Source: CAD feature listing. Evaluate the final solid. Frame: model axes, mm. Give positions to 0.01 mm unless a question says otherwise; leave off trailing zeros. Write each loop counter-clockwise with the first axis right and the second up, starting at its lowest first coordinate (ties: lowest second). Pieces come first, ordered by that corner, then holes. Notation, with made-up numbers: (2.25, 28) -> (57.25, 28) arc R20 ccw to (57.25, 58) -> close; hole circle Ø11 at (89, 77). An arc over 180 degrees is marked (long way). Use one line per item in the form item = value. Start each with the question number.
(1) First-contact query: P1, Ø2, axis at x = 12.5, y = 18.5, coming from the -Z side. Flat tip, straight axial feed; report the tip coordinate or a pass-through.
(2) Cut plane B-B, the plane y = 19.1. Output: boundary loops of the cut face in (x, z).
(3) Material intervals for line 1 along Z through (x, y) = (31, 19.1); line 2 along Z through (x, y) = (39, 17.95); line 3 along X through (y, z) = (17.15, 29), sorted ascending. Write a range as from..to.
(4) Cut plane C-C, the plane z = 13. Output: boundary loops of the cut face in (x, y).
(5) Cut plane D-D, the plane z = 24.5. Output: boundary loops of the cut face in (x, y), and give its area (3 significant figures).
(6) Cut plane A-A, the plane x = 31. Output: boundary loops of the cut face in (y, z), and give its area (3 significant figures).
(7) Draft query along Z for faces 1 (the face through (14, 20, 8)), 2 (the face through (36.802, 17.972, 3.903)), 3 (the face through (7.497, 17.972, 37.787)). Return one class per face: pulls with the +Z half, pulls with the -Z half, needs draft (parallel to the pull), parting line crosses it, or undercut.
from build123d import *

# Parameters (mm, degrees)
CYLINDER019_R          = 2.2
CYLINDER019_DEPTH      = 26
CYLINDER019_ROLL_ANGLE = -90
ARRAY005_X_COUNT       = 2
ARRAY005_X_PITCH       = 8
ARRAY005_Z_COUNT       = 2
ARRAY005_Z_PITCH       = 9
CYLINDER018_R          = 30
CYLINDER018_DEPTH      = 4
CYLINDER018_ROLL_ANGLE = -90


with BuildPart() as obj1:
    # Cylinder019 → Cylinder019 (new body)
    with BuildSketch(Plane.XY):
        Circle(CYLINDER019_R)
    extrude(amount=CYLINDER019_DEPTH)


with BuildPart() as obj1_1:
    # Cylinder019 roll: moved
    add(obj1.part.rotate(Axis((0, 0, 0), (1, 0, 0)), CYLINDER019_ROLL_ANGLE))


with BuildPart() as obj1_2:
    # Cylinder019 placement: moved
    add(obj1_1.part.moved(Location((202, 0, 4))))

    # Array005 X: obj1_2


with BuildPart() as obj1_3:
    add(obj1_2.part)
    with Locations(*[(i * ARRAY005_X_PITCH, 0, 0) for i in range(1, ARRAY005_X_COUNT)]):
        add(obj1_2.part)

    # Array005 Z: obj1_2


with BuildPart() as obj1_4:
    add(obj1_3.part)
    with Locations(*[(0, 0, i * ARRAY005_Z_PITCH) for i in range(1, ARRAY005_Z_COUNT)]):
        add(obj1_3.part)


with BuildPart() as obj2:
    # Cylinder018 → Cylinder018 (new body)
    with BuildSketch(Plane.XY):
        Circle(CYLINDER018_R)
    extrude(amount=CYLINDER018_DEPTH)


with BuildPart() as obj2_1:
    # Cylinder018 roll: moved
    add(obj2.part.rotate(Axis((0, 0, 0), (1, 0, 0)), CYLINDER018_ROLL_ANGLE))


with BuildPart() as obj2_2:
    # Cylinder018 placement: moved
    add(obj2_1.part.moved(Location((185, 20, 8.5))))

    # Cut015: cut obj1
    add(obj1_4.part, mode=Mode.SUBTRACT)


with BuildPart() as obj2_3:
    # Cut015 placement: moved
    add(obj2_2.part.moved(Location((-171, -4, 0))))


solid = obj2_3.part
Geometry says:
q1.P1 = -21.5
q2.outline = circle Ø60 at (14, 8.5); hole circle Ø4.4 at (31, 4); hole circle Ø4.4 at (31, 13); hole circle Ø4.4 at (39, 4); hole circle Ø4.4 at (39, 13)
q3.line_1 = -16.22..1.8, 6.2..10.8, 15.2..33.22
q3.line_2 = -8.08..1.8, 6.2..10.8, 15.2..25.08
q3.line_3 = -7.9..35.9
q4.outline = (-15.66, 16) -> (28.8, 16) -> (28.8, 20) -> (-15.66, 20) -> close; (33.2, 16) -> (36.8, 16) -> (36.8, 20) -> (33.2, 20) -> close; (41.2, 16) -> (43.66, 16) -> (43.66, 20) -> (41.2, 20) -> close
q5.outline = (-11.38, 16) -> (39.38, 16) -> (39.38, 20) -> (-11.38, 20) -> close
q5.area = 203 mm^2
q6.outline = (16, -16.22) -> (20, -16.22) -> (20, 1.8) -> (16, 1.8) -> close; (16, 6.2) -> (20, 6.2) -> (20, 10.8) -> (16, 10.8) -> close; (16, 15.2) -> (20, 15.2) -> (20, 33.22) -> (16, 33.22) -> close
q6.area = 163 mm^2
q7.face_1 = needs draft
q7.face_2 = undercut
q7.face_3 = parting line crosses it
